For this review, use the dimensioned drawing (mm, ordinates from the lowest corner) and the shaded views. A direction names the side the tool comes from. Give positions to 0.01 mm unless a question says otherwise; leave off trailing zeros. Order: outer loops, then holes, each group sorted by start corner. A loop starts at its lowest first (then second) coordinate and runs counter-clockwise, first axis right, second up. Notation, with made-up numbers: (55, -29.75) - (67, -29.75) arc R17 cw to (67, -2.75) - close; hole circle Ø11 at (57, 18.5). An arc over 180 degrees is marked (long way). Use a Markdown table: item, result. Add a question column.
1) We need section D-D on x = 14. Write out the cut boundary in (y, z), then the cut area to 3 significant figures.
2) Wall thickness on L1, parallel to X at y = 25, z = 5.5; L2, parallel to Y at x = 14, z = 12.65; L3, parallel to Y at x = 48, z = 1.75: over which ranges is each line inside the solid? List them lowest first.
3) We need section C-C on y = 27.5. Write out the cut boundary in (x, z).
4) Machinability: for the marked faces 1, 2 and 3, which of the approach directions +Z, -Z, +X, -X, +Y, -Y give a long, thin tool a straight path to every point of the face, cutting with its end or side? Answer none if there is none.
5) We need section B-B on z = 3. Write out the cut boundary in (x, y).
6) We need section A-A on x = 36.5. Write out the cut boundary in (y, z).
7) Clearance check with flat-ended pins moving along their axes: P1, Ø3, axis at x = 30.5, z = 4, coming from the -Y side; P2, Ø2, axis at x = 13.5, y = 46.5, coming from the +Z side; P3, Ø6, axis at x = 29, y = 47.5, coming from the -Z side; P4, Ø5, axis at y = 22.5, z = 16, coming from the +X side. State where each tip first meets the part, or that it passes through.
8) Mouldability with a two-part tool opening along X and no side actions: class the marked faces 4, 5, 6 and 7 as released by +X, released by -X, zero draft, split by the parting line, or undercut.
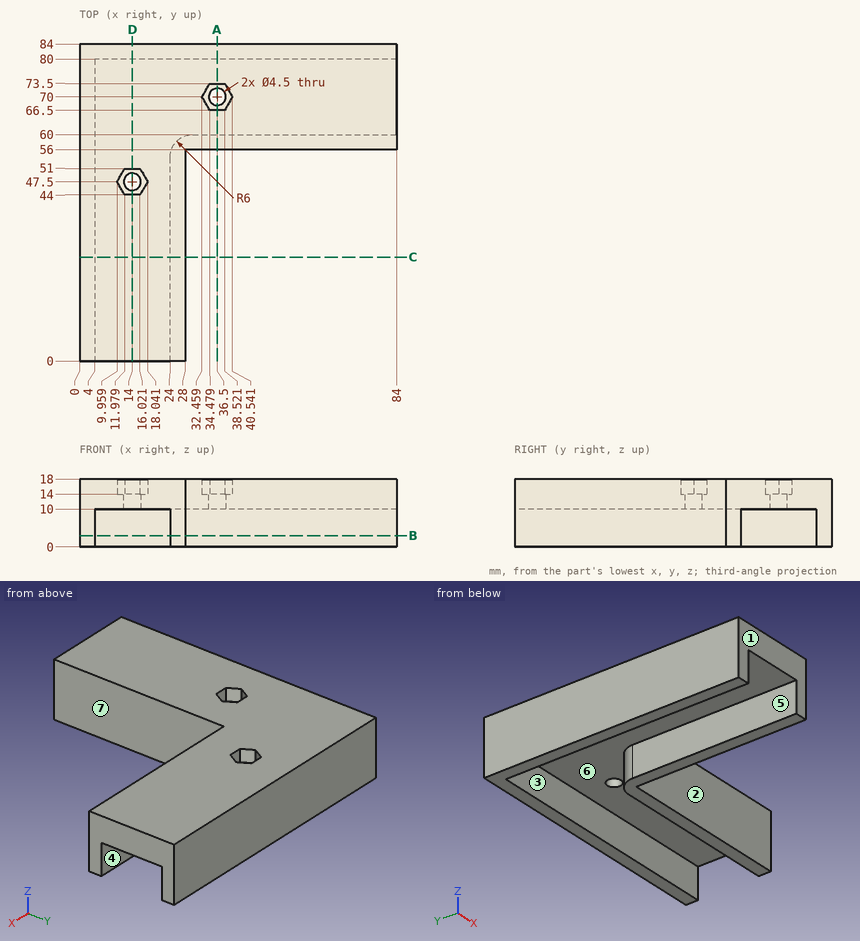
Checked values:
| question | item | result |
|---|---|---|
| 1 | outline | (0, 10) - (45.25, 10) - (45.25, 14) - (44, 14) - (44, 18) - (0, 18) - close; (49.75, 10) - (80, 10) - (80, 0) - (84, 0) - (84, 18) - (51, 18) - (51, 14) - (49.75, 14) - close |
| 1 | area | 666 mm² |
| 2 | L1 | 0 to 4, 24 to 28 |
| 2 | L2 | 0 to 45.25, 49.75 to 84 |
| 2 | L3 | 56 to 60, 80 to 84 |
| 3 | outline | (0, 0) - (4, 0) - (4, 10) - (24, 10) - (24, 0) - (28, 0) - (28, 18) - (0, 18) - close |
| 4 | face 1 | +Z, -Z, +X, -X, -Y |
| 4 | face 2 | +Z, -Z, +X, -Y |
| 4 | face 3 | -Z, +X |
| 5 | outline | (0, 0) - (4, 0) - (4, 80) - (84, 80) - (84, 84) - (0, 84) - close; (24, 0) - (28, 0) - (28, 56) - (84, 56) - (84, 60) - (30, 60) arc R6 ccw to (24, 54) - close |
| 6 | outline | (56, 0) - (60, 0) - (60, 10) - (67.75, 10) - (67.75, 14) - (66.5, 14) - (66.5, 18) - (56, 18) - close; (72.25, 10) - (80, 10) - (80, 0) - (84, 0) - (84, 18) - (73.5, 18) - (73.5, 14) - (72.25, 14) - close |
| 7 | P1 | y = 56 |
| 7 | P2 | through |
| 7 | P3 | z = 0 |
| 7 | P4 | x = 28 |
| 8 | face 4 | zero draft |
| 8 | face 5 | undercut |
| 8 | face 6 | undercut |
| 8 | face 7 | released by +X |
